from build123d import *

# Parameters (mm, degrees)
F0_W    = 18.5
F0_H    = 17
F2_SIZE = 2
F3_SIZE = 1


with BuildPart() as f1:
    # F0 (on Front) → F1 (revolve)
    with BuildSketch(Plane.XZ):
        with Locations((26.75, 8.5)):
            Rectangle(F0_W, F0_H)
    revolve(axis=Axis((0, 0, 7.291329), (0, 0, 1)))

    # F2
    f2_edges = [f1.edges().sort_by_distance(p)[0] for p in [
        (-36, 0, 17),
        (-36, 0, 0),
        (36, 0, 8.5),
    ]]
    chamfer(f2_edges, length=F2_SIZE)

    # F3
    f3_edges = [f1.edges().sort_by_distance(p)[0] for p in [
        (-17.5, 0, 17),
        (-17.5, 0, 0),
    ]]
    chamfer(f3_edges, length=F3_SIZE)


solid = f1.part
Design review of the part built by this model. Coordinates are the model's own, in mm. Give positions to 0.01 mm unless a question says otherwise; leave off trailing zeros. Write each loop counter-clockwise with the first axis right and the second up, starting at its lowest first coordinate (ties: lowest second). Pieces come first, ordered by that corner, then holes. Notation, with made-up numbers: M 38,77 L 77,77 A34 cw 77,107 Z; hole C 10,69 d2. An arc over 180 degrees is marked long. Answer as a JSON object with one key per item and string values. Group by question number.
1) Clearance check with flat-ended pins moving along their axes: pin 1 Ø2 at (y, z) = (3, 2) entering from -X; pin 2 Ø10 at (y, z) = (27, 13) entering from -X; pin 3 Ø5 at (x, z) = (-19.5, 13.5) entering from +Y; pin 4 Ø10 at (y, z) = (-3.5, 8.5) entering from -X. State where each tip first meets the part, or that it passes through.
2) We need section C-C (z = 11.75). Give the boundary of the cut face in (x, y).
3) We need section A-A (x = 0). Give the boundary of the cut face in (y, z).
4) For line 1 along Y through (x, z) = (0, 5.75); line 2 along Y through (x, z) = (-5, 9.5); line 3 along X through (y, z) = (-3, 12.75), list the stretches that pass through material, from the lowest coordinate up.
5) Mouldability with a two-part tool opening along X and no side actions: class faces 1 (the face through (-15, -15, 17)), 2 (the face through (-4.686, 35.694, 8.591)), 3 (the face through (-13.887, -10.648, 8.605)) as released by +X, released by -X, zero draft, split by the parting line, or undercut.
Answer key:
{
 "1": {"pin 1": "stops at x = -35.94", "pin 2": "stops at x = -28.5", "pin 3": "stops at y = 31.73", "pin 4": "stops at x = -36"},
 "2": {"outline": "C 0,0 d72; hole C 0,0 d35"},
 "3": {"outline": "M -36,2 L -34,0 L -18.5,0 L -17.5,1 L -17.5,16 L -18.5,17 L -34,17 L -36,15 Z; M 17.5,1 L 18.5,0 L 34,0 L 36,2 L 36,15 L 34,17 L 18.5,17 L 17.5,16 Z"},
 "4": {"line 1": "y = -36 to -17.5, 17.5 to 36", "line 2": "y = -35.65 to -16.77, 16.77 to 35.65", "line 3": "x = -35.87 to -17.24, 17.24 to 35.87"},
 "5": {"face 1": "zero draft", "face 2": "split by the parting line", "face 3": "undercut"}
}
